Verification items for the finished model (mm, model axes). Give positions to 0.01 mm unless a question says otherwise; leave off trailing zeros. Order: outer loops, then holes, each group sorted by start corner. A loop starts at its lowest first (then second) coordinate and runs counter-clockwise, first axis right, second up.
(1) Scan lines: L1, parallel to Y at x = 1.5, z = 0.85; L2, parallel to Y at x = 6, z = 0.4; L3, parallel to X at y = -20.5, z = 0.45. Record each from-to range of solid material in increasing order.
(2) Sectioned sample at A-A on x = -2. Record the cut outline in (y, z).
(3) Sectioned sample at B-B on z = 1.1. Record the cut outline in (x, y), plus the area to 3 significant figures.
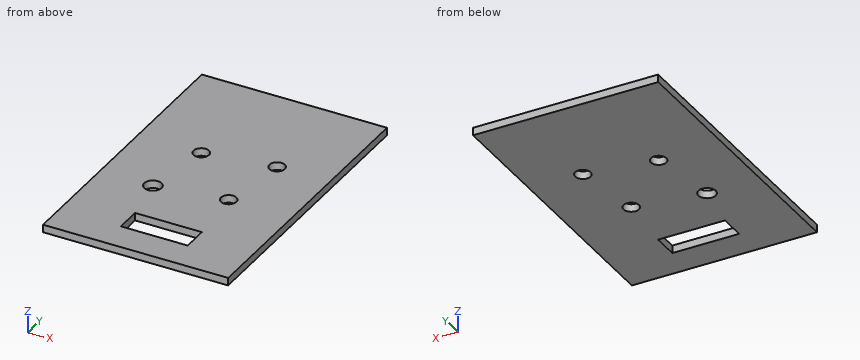
```python
from build123d import *

# Parameters (mm, degrees)
SKETCH1_R           = 1.5
SKETCH1_R_2         = 1.680409227
SKETCH1_W           = 13
SKETCH1_H           = 5
BOSS_EXTRUDE3_DEPTH = 1.5


with BuildPart() as part:
    # Sketch1 → Boss-Extrude3 (new body)
    with BuildSketch(Plane.XY):
        Polygon((-18, 0), (-18, 28), (18, 28), (18, -28), (-18, -28), align=None)
        with Locations((7.778174593, 7.778174593)):
            Circle(SKETCH1_R, mode=Mode.SUBTRACT)
        with Locations((-5.73801436, 5.574512642)):
            Circle(SKETCH1_R, mode=Mode.SUBTRACT)
        with Locations((-7.778174593, -7.778174593)):
            Circle(SKETCH1_R_2, mode=Mode.SUBTRACT)
        with Locations((5.73801436, -5.574512642)):
            Circle(SKETCH1_R, mode=Mode.SUBTRACT)
        with Locations((0.358519309, -19.559341262)):
            Rectangle(SKETCH1_W, SKETCH1_H, mode=Mode.SUBTRACT)
    extrude(amount=BOSS_EXTRUDE3_DEPTH)


solid = part.part
```
Ans:
1. L1: y = -28 to -22.06, -17.06 to 28
1. L2: y = -28 to -22.06, -17.06 to -7.05, -4.1 to 28
1. L3: x = -18 to -6.14, 6.86 to 18
2. outline: (-28, 0) - (-22.06, 0) - (-22.06, 1.5) - (-28, 1.5) - close; (-17.06, 0) - (28, 0) - (28, 1.5) - (-17.06, 1.5) - close
3. outline: (-18, -28) - (18, -28) - (18, 28) - (-18, 28) - close; hole circle Ø3.36 at (-7.78, -7.78); hole circle Ø3 at (-5.74, 5.57); hole (-6.14, -22.06) - (6.86, -22.06) - (6.86, -17.06) - (-6.14, -17.06) - close; hole circle Ø3 at (5.74, -5.57); hole circle Ø3 at (7.78, 7.78)
3. area: 1,920 mm2
